```python
from build123d import *

# Parameters (mm, degrees)
BLANKSKE_W                      = 150
BLANKSKE_H                      = 12
BLANK_DEPTH                     = 5
TOOTHCUTSIM_DEPTH               = 151.562279473
TEETHCUTS_COUNT                 = 25
TEETHCUTS_PITCH                 = 6.2831853
SKETCH1_W                       = 150
SKETCH1_H                       = 6
BOSS_EXTRUDE1_DEPTH             = 10
MIRROR1_COPY_1_DEPTH            = 151.562279473
MIRROR1_COPY_2_DEPTH            = 151.562279473
MIRROR1_COPY_3_DEPTH            = 151.562279473
MIRROR1_COPY_4_DEPTH            = 151.562279473
MIRROR1_COPY_5_DEPTH            = 151.562279473
MIRROR1_COPY_6_DEPTH            = 151.562279473
MIRROR1_COPY_7_DEPTH            = 151.562279473
MIRROR1_COPY_8_DEPTH            = 151.562279473
MIRROR1_COPY_9_DEPTH            = 151.562279473
MIRROR1_COPY_10_DEPTH           = 151.562279473
MIRROR1_COPY_11_DEPTH           = 151.562279473
MIRROR1_COPY_12_DEPTH           = 151.562279473
MIRROR1_COPY_13_DEPTH           = 151.562279473
MIRROR1_COPY_14_DEPTH           = 151.562279473
MIRROR1_COPY_15_DEPTH           = 151.562279473
MIRROR1_COPY_16_DEPTH           = 151.562279473
MIRROR1_COPY_17_DEPTH           = 151.562279473
MIRROR1_COPY_18_DEPTH           = 151.562279473
MIRROR1_COPY_19_DEPTH           = 151.562279473
MIRROR1_COPY_20_DEPTH           = 151.562279473
MIRROR1_COPY_21_DEPTH           = 151.562279473
MIRROR1_COPY_22_DEPTH           = 151.562279473
MIRROR1_COPY_23_DEPTH           = 151.562279473
MIRROR1_COPY_24_DEPTH           = 151.562279473
MIRROR1_COPY_25_DEPTH           = 151.562279473
F_4_0MM_DOWEL_HOLE1_D           = 4
F_4_0MM_DOWEL_HOLE1_DEPTH       = 3
F_4_0MM_DOWEL_HOLE1_CSINK_D     = 4.05
F_4_0MM_DOWEL_HOLE1_CSINK_ANGLE = 90
F_4_0MM_DOWEL_HOLE1_TIP         = 1.201721238
SKETCH7_W                       = 12
SKETCH7_H                       = 6
CUT_EXTRUDE1_DEPTH              = 9.2
FILLET2_R                       = 5
FILLET3_R                       = 5


with BuildPart() as part:
    # BlankSke → Blank (new body)
    with BuildSketch(Plane.XY):
        with Locations((75, 6)):
            Rectangle(BLANKSKE_W, BLANKSKE_H)
    blank = extrude(amount=-BLANK_DEPTH)

    # TooCutSkeSim → ToothCutSim (cut, through all)
    with BuildSketch(Plane.XY):
        Polygon((0.861870739, 7.5), (-0.861870739, 7.5), (-2.508981637, 12.0254), (2.508981637, 12.0254), align=None)
    toothcutsim = extrude(amount=-TOOTHCUTSIM_DEPTH, mode=Mode.SUBTRACT)

    # TeethCuts: ToothCutSim ×25
    with Locations(*[(i * TEETHCUTS_PITCH, 0, 0) for i in range(1, TEETHCUTS_COUNT)]):
        add(toothcutsim, mode=Mode.SUBTRACT)

    # Sketch1 → Boss-Extrude1 (add)
    with BuildSketch(Plane(origin=(0, 0, -5), x_dir=(-1, 0, 0), z_dir=(0, 0, -1))):
        with Locations((-75, -3)):
            Rectangle(SKETCH1_W, SKETCH1_H)
    extrude(amount=-BOSS_EXTRUDE1_DEPTH)

    # Mirror1: Blank across plane
    add(blank.mirror(Plane.XY))

    # Mirror1 copy 1 sketch → Mirror1 copy 1 (cut, through all)
    with BuildSketch(Plane(origin=(6.2831853, 0, 0), x_dir=(1, 0, 0), z_dir=(0, 0, -1))):
        Polygon((0.861870739, -7.5), (-0.861870739, -7.5), (-2.508981637, -12.0254), (2.508981637, -12.0254), align=None)
    extrude(amount=-MIRROR1_COPY_1_DEPTH, mode=Mode.SUBTRACT)

    # Mirror1 copy 2 sketch → Mirror1 copy 2 (cut, through all)
    with BuildSketch(Plane(origin=(12.5663706, 0, 0), x_dir=(1, 0, 0), z_dir=(0, 0, -1))):
        Polygon((0.861870739, -7.5), (-0.861870739, -7.5), (-2.508981637, -12.0254), (2.508981637, -12.0254), align=None)
    extrude(amount=-MIRROR1_COPY_2_DEPTH, mode=Mode.SUBTRACT)

    # Mirror1 copy 3 sketch → Mirror1 copy 3 (cut, through all)
    with BuildSketch(Plane(origin=(18.8495559, 0, 0), x_dir=(1, 0, 0), z_dir=(0, 0, -1))):
        Polygon((0.861870739, -7.5), (-0.861870739, -7.5), (-2.508981637, -12.0254), (2.508981637, -12.0254), align=None)
    extrude(amount=-MIRROR1_COPY_3_DEPTH, mode=Mode.SUBTRACT)

    # Mirror1 copy 4 sketch → Mirror1 copy 4 (cut, through all)
    with BuildSketch(Plane(origin=(25.1327412, 0, 0), x_dir=(1, 0, 0), z_dir=(0, 0, -1))):
        Polygon((0.861870739, -7.5), (-0.861870739, -7.5), (-2.508981637, -12.0254), (2.508981637, -12.0254), align=None)
    extrude(amount=-MIRROR1_COPY_4_DEPTH, mode=Mode.SUBTRACT)

    # Mirror1 copy 5 sketch → Mirror1 copy 5 (cut, through all)
    with BuildSketch(Plane(origin=(31.4159265, 0, 0), x_dir=(1, 0, 0), z_dir=(0, 0, -1))):
        Polygon((0.861870739, -7.5), (-0.861870739, -7.5), (-2.508981637, -12.0254), (2.508981637, -12.0254), align=None)
    extrude(amount=-MIRROR1_COPY_5_DEPTH, mode=Mode.SUBTRACT)

    # Mirror1 copy 6 sketch → Mirror1 copy 6 (cut, through all)
    with BuildSketch(Plane(origin=(37.6991118, 0, 0), x_dir=(1, 0, 0), z_dir=(0, 0, -1))):
        Polygon((0.861870739, -7.5), (-0.861870739, -7.5), (-2.508981637, -12.0254), (2.508981637, -12.0254), align=None)
    extrude(amount=-MIRROR1_COPY_6_DEPTH, mode=Mode.SUBTRACT)

    # Mirror1 copy 7 sketch → Mirror1 copy 7 (cut, through all)
    with BuildSketch(Plane(origin=(43.9822971, 0, 0), x_dir=(1, 0, 0), z_dir=(0, 0, -1))):
        Polygon((0.861870739, -7.5), (-0.861870739, -7.5), (-2.508981637, -12.0254), (2.508981637, -12.0254), align=None)
    extrude(amount=-MIRROR1_COPY_7_DEPTH, mode=Mode.SUBTRACT)

    # Mirror1 copy 8 sketch → Mirror1 copy 8 (cut, through all)
    with BuildSketch(Plane(origin=(50.2654824, 0, 0), x_dir=(1, 0, 0), z_dir=(0, 0, -1))):
        Polygon((0.861870739, -7.5), (-0.861870739, -7.5), (-2.508981637, -12.0254), (2.508981637, -12.0254), align=None)
    extrude(amount=-MIRROR1_COPY_8_DEPTH, mode=Mode.SUBTRACT)

    # Mirror1 copy 9 sketch → Mirror1 copy 9 (cut, through all)
    with BuildSketch(Plane(origin=(56.5486677, 0, 0), x_dir=(1, 0, 0), z_dir=(0, 0, -1))):
        Polygon((0.861870739, -7.5), (-0.861870739, -7.5), (-2.508981637, -12.0254), (2.508981637, -12.0254), align=None)
    extrude(amount=-MIRROR1_COPY_9_DEPTH, mode=Mode.SUBTRACT)

    # Mirror1 copy 10 sketch → Mirror1 copy 10 (cut, through all)
    with BuildSketch(Plane(origin=(62.831853, 0, 0), x_dir=(1, 0, 0), z_dir=(0, 0, -1))):
        Polygon((0.861870739, -7.5), (-0.861870739, -7.5), (-2.508981637, -12.0254), (2.508981637, -12.0254), align=None)
    extrude(amount=-MIRROR1_COPY_10_DEPTH, mode=Mode.SUBTRACT)

    # Mirror1 copy 11 sketch → Mirror1 copy 11 (cut, through all)
    with BuildSketch(Plane(origin=(69.1150383, 0, 0), x_dir=(1, 0, 0), z_dir=(0, 0, -1))):
        Polygon((0.861870739, -7.5), (-0.861870739, -7.5), (-2.508981637, -12.0254), (2.508981637, -12.0254), align=None)
    extrude(amount=-MIRROR1_COPY_11_DEPTH, mode=Mode.SUBTRACT)

    # Mirror1 copy 12 sketch → Mirror1 copy 12 (cut, through all)
    with BuildSketch(Plane(origin=(75.3982236, 0, 0), x_dir=(1, 0, 0), z_dir=(0, 0, -1))):
        Polygon((0.861870739, -7.5), (-0.861870739, -7.5), (-2.508981637, -12.0254), (2.508981637, -12.0254), align=None)
    extrude(amount=-MIRROR1_COPY_12_DEPTH, mode=Mode.SUBTRACT)

    # Mirror1 copy 13 sketch → Mirror1 copy 13 (cut, through all)
    with BuildSketch(Plane(origin=(81.6814089, 0, 0), x_dir=(1, 0, 0), z_dir=(0, 0, -1))):
        Polygon((0.861870739, -7.5), (-0.861870739, -7.5), (-2.508981637, -12.0254), (2.508981637, -12.0254), align=None)
    extrude(amount=-MIRROR1_COPY_13_DEPTH, mode=Mode.SUBTRACT)

    # Mirror1 copy 14 sketch → Mirror1 copy 14 (cut, through all)
    with BuildSketch(Plane(origin=(87.9645942, 0, 0), x_dir=(1, 0, 0), z_dir=(0, 0, -1))):
        Polygon((0.861870739, -7.5), (-0.861870739, -7.5), (-2.508981637, -12.0254), (2.508981637, -12.0254), align=None)
    extrude(amount=-MIRROR1_COPY_14_DEPTH, mode=Mode.SUBTRACT)

    # Mirror1 copy 15 sketch → Mirror1 copy 15 (cut, through all)
    with BuildSketch(Plane(origin=(94.2477795, 0, 0), x_dir=(1, 0, 0), z_dir=(0, 0, -1))):
        Polygon((0.861870739, -7.5), (-0.861870739, -7.5), (-2.508981637, -12.0254), (2.508981637, -12.0254), align=None)
    extrude(amount=-MIRROR1_COPY_15_DEPTH, mode=Mode.SUBTRACT)

    # Mirror1 copy 16 sketch → Mirror1 copy 16 (cut, through all)
    with BuildSketch(Plane(origin=(100.5309648, 0, 0), x_dir=(1, 0, 0), z_dir=(0, 0, -1))):
        Polygon((0.861870739, -7.5), (-0.861870739, -7.5), (-2.508981637, -12.0254), (2.508981637, -12.0254), align=None)
    extrude(amount=-MIRROR1_COPY_16_DEPTH, mode=Mode.SUBTRACT)

    # Mirror1 copy 17 sketch → Mirror1 copy 17 (cut, through all)
    with BuildSketch(Plane(origin=(106.8141501, 0, 0), x_dir=(1, 0, 0), z_dir=(0, 0, -1))):
        Polygon((0.861870739, -7.5), (-0.861870739, -7.5), (-2.508981637, -12.0254), (2.508981637, -12.0254), align=None)
    extrude(amount=-MIRROR1_COPY_17_DEPTH, mode=Mode.SUBTRACT)

    # Mirror1 copy 18 sketch → Mirror1 copy 18 (cut, through all)
    with BuildSketch(Plane(origin=(113.0973354, 0, 0), x_dir=(1, 0, 0), z_dir=(0, 0, -1))):
        Polygon((0.861870739, -7.5), (-0.861870739, -7.5), (-2.508981637, -12.0254), (2.508981637, -12.0254), align=None)
    extrude(amount=-MIRROR1_COPY_18_DEPTH, mode=Mode.SUBTRACT)

    # Mirror1 copy 19 sketch → Mirror1 copy 19 (cut, through all)
    with BuildSketch(Plane(origin=(119.3805207, 0, 0), x_dir=(1, 0, 0), z_dir=(0, 0, -1))):
        Polygon((0.861870739, -7.5), (-0.861870739, -7.5), (-2.508981637, -12.0254), (2.508981637, -12.0254), align=None)
    extrude(amount=-MIRROR1_COPY_19_DEPTH, mode=Mode.SUBTRACT)

    # Mirror1 copy 20 sketch → Mirror1 copy 20 (cut, through all)
    with BuildSketch(Plane(origin=(125.663706, 0, 0), x_dir=(1, 0, 0), z_dir=(0, 0, -1))):
        Polygon((0.861870739, -7.5), (-0.861870739, -7.5), (-2.508981637, -12.0254), (2.508981637, -12.0254), align=None)
    extrude(amount=-MIRROR1_COPY_20_DEPTH, mode=Mode.SUBTRACT)

    # Mirror1 copy 21 sketch → Mirror1 copy 21 (cut, through all)
    with BuildSketch(Plane(origin=(131.9468913, 0, 0), x_dir=(1, 0, 0), z_dir=(0, 0, -1))):
        Polygon((0.861870739, -7.5), (-0.861870739, -7.5), (-2.508981637, -12.0254), (2.508981637, -12.0254), align=None)
    extrude(amount=-MIRROR1_COPY_21_DEPTH, mode=Mode.SUBTRACT)

    # Mirror1 copy 22 sketch → Mirror1 copy 22 (cut, through all)
    with BuildSketch(Plane(origin=(138.2300766, 0, 0), x_dir=(1, 0, 0), z_dir=(0, 0, -1))):
        Polygon((0.861870739, -7.5), (-0.861870739, -7.5), (-2.508981637, -12.0254), (2.508981637, -12.0254), align=None)
    extrude(amount=-MIRROR1_COPY_22_DEPTH, mode=Mode.SUBTRACT)

    # Mirror1 copy 23 sketch → Mirror1 copy 23 (cut, through all)
    with BuildSketch(Plane(origin=(144.5132619, 0, 0), x_dir=(1, 0, 0), z_dir=(0, 0, -1))):
        Polygon((0.861870739, -7.5), (-0.861870739, -7.5), (-2.508981637, -12.0254), (2.508981637, -12.0254), align=None)
    extrude(amount=-MIRROR1_COPY_23_DEPTH, mode=Mode.SUBTRACT)

    # Mirror1 copy 24 sketch → Mirror1 copy 24 (cut, through all)
    with BuildSketch(Plane(origin=(150.7964472, 0, 0), x_dir=(1, 0, 0), z_dir=(0, 0, -1))):
        Polygon((0.861870739, -7.5), (-0.861870739, -7.5), (-2.508981637, -12.0254), (2.508981637, -12.0254), align=None)
    extrude(amount=-MIRROR1_COPY_24_DEPTH, mode=Mode.SUBTRACT)

    # Mirror1 copy 25 sketch → Mirror1 copy 25 (cut, through all)
    with BuildSketch(Plane(origin=(0, 0, 0), x_dir=(1, 0, 0), z_dir=(0, 0, -1))):
        Polygon((0.861870739, -7.5), (-0.861870739, -7.5), (-2.508981637, -12.0254), (2.508981637, -12.0254), align=None)
    extrude(amount=-MIRROR1_COPY_25_DEPTH, mode=Mode.SUBTRACT)

    # Ø4.0mm Dowel Hole1
    with Locations(Plane(origin=(0, -6, 0), x_dir=(-1, 0, 0), z_dir=(0, -1, 0))):
        with Locations((-50, 0), (-100, 0)):
            CounterSinkHole(F_4_0MM_DOWEL_HOLE1_D / 2, F_4_0MM_DOWEL_HOLE1_CSINK_D / 2, depth=F_4_0MM_DOWEL_HOLE1_DEPTH, counter_sink_angle=F_4_0MM_DOWEL_HOLE1_CSINK_ANGLE)
            with Locations((0, 0, -(F_4_0MM_DOWEL_HOLE1_DEPTH + F_4_0MM_DOWEL_HOLE1_TIP / 2))):  # 118° drill point
                Cone(0, F_4_0MM_DOWEL_HOLE1_D / 2, F_4_0MM_DOWEL_HOLE1_TIP, mode=Mode.SUBTRACT)

    # Sketch7 → Cut-Extrude1 (cut)
    with BuildSketch(Plane(origin=(0, 0, -5), x_dir=(-1, 0, 0), z_dir=(0, 0, -1))):
        Polygon((-106, -3), (-100, -3), (-94, -3), (-94, 3), (-106, 3), align=None)
        with Locations((-50, 0)):
            Rectangle(SKETCH7_W, SKETCH7_H)
    extrude(amount=-CUT_EXTRUDE1_DEPTH, mode=Mode.SUBTRACT)

    # Fillet2
    fillet2_edges = [part.edges().sort_by_distance(p)[0] for p in [
        (106, 3, -0.4),
        (94, 3, -0.4),
    ]]
    fillet(fillet2_edges, radius=FILLET2_R)

    # Fillet3
    fillet3_edges = [part.edges().sort_by_distance(p)[0] for p in [
        (56, 3, -0.4),
        (44, 3, -0.4),
    ]]
    fillet(fillet3_edges, radius=FILLET3_R)


solid = part.part
```
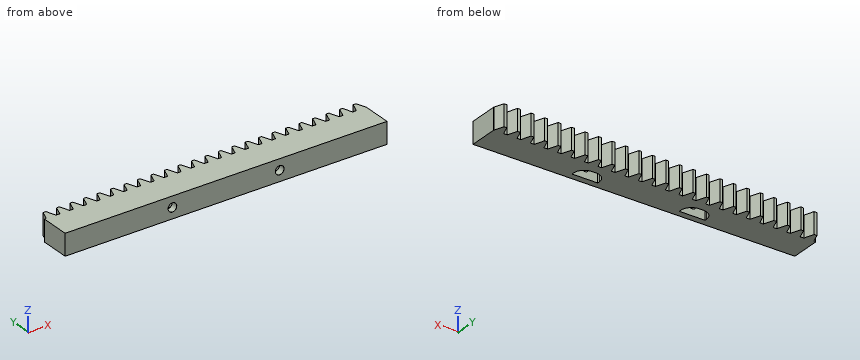
Part model, mm, in its own coordinate system. Give positions to 0.01 mm unless a question says otherwise; leave off trailing zeros. Order: outer loops, then holes, each group sorted by start corner. A loop starts at its lowest first (then second) coordinate and runs counter-clockwise, first axis right, second up. Notation, with made-up numbers: (13.5, -10) - (66.5, -10) arc R19 ccw to (66.5, -3) - close; hole circle Ø6 at (-26, 81.25). An arc over 180 degrees is marked (long way). Use one line per item in the form item = value.
Item 1: Pin check, flat tips, straight feed: pin 1 Ø4 at (y, z) = (2.5, 2) entering from -X; pin 2 Ø2 at (x, z) = (100, 0) entering from -Y; pin 3 Ø0.9 at (x, z) = (50.5, 1) entering from +Y. Stop position of each tip, or through.
Solution:
pin_1 = 0
pin_2 = 3
pin_3 = 7.5
Item 2: Slice it at A-A on y = 10.5. Count the separate pieces of the cut face and the enclosed holes in it, and give its area (3 significant figures).
Solution:
separate_pieces = 24
enclosed_holes = 0
area = 570 mm2
Item 3: Slice it at B-B on y = 0. Give the cut face in (x, z), and give its area (3 significant figures).
Solution:
outline = (0, -5) - (44.42, -5) - (44.42, 4.2) - (55.58, 4.2) - (55.58, -5) - (94.42, -5) - (94.42, 4.2) - (105.58, 4.2) - (105.58, -5) - (150, -5) - (150, 5) - (0, 5) - close
area = 1,290 mm2
Item 4: Probe probe 1 along X at (y, z) = (-2.25, 1.75); probe 2 along Z at (x, y) = (100, -4); probe 3 along X at (y, z) = (-0.75, 0.25). List the from-to ranges inside material, lowest first. Write a range as from..to.
Solution:
probe_1 = 0..44, 56..94, 106..150
probe_2 = -5..-2, 2..5
probe_3 = 0..44.16, 55.84..94.16, 105.84..150
